Geometry: see drawing. Coordinates: mm, zero at the bounding-box minimum. Round coordinates to 2 decimals unless told otherwise and drop trailing zeros. Order: outer loops, then holes, each group sorted by start corner. A loop starts at its lowest first (then second) coordinate and runs counter-clockwise, first axis right, second up. Notation, with made-up numbers: (-26.75, -22) - (-1.75, -22) arc R26 ccw to (-1.75, 2) - close; hole circle Ø6 at (38.25, -26). An arc over 180 degrees is marked (long way). Put each result on its own line as item: value. Start each with the question number.
1) Contact query for flat-ended pins moving along their axis: P1, Ø4, axis at y = 43.5, z = 1.5, coming from the -X side; P2, Ø1, axis at y = 7.5, z = 4, coming from the -X side. Output: stop coordinate, or through.
2) Section A-A on x = 6.75. Output: boundary loops of the cut face in (y, z), then the cut area to 3 significant figures.
3) Section B-B on z = 4. Output: boundary loops of the cut face in (x, y).
4) Section C-C on y = 27. Output: boundary loops of the cut face in (x, z).
5) Line query: probe 1 along Y at (x, z) = (8.75, 7.75); probe 2 along Z at (x, y) = (2.5, 19); probe 3 along X at (y, z) = (12, 2.75). Output: solid intervals per line, ascending. Write a range as [from, to].
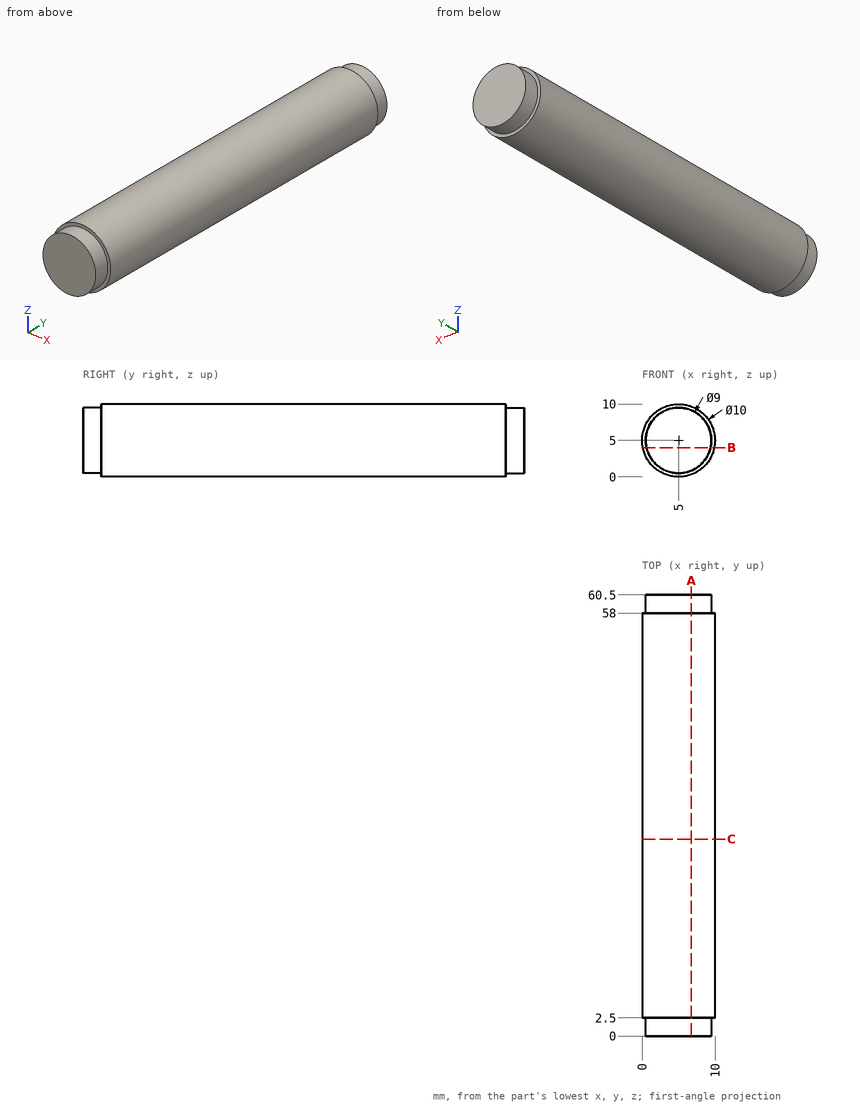
Answer sheet:
1. P1: x = 0.23
1. P2: x = 0.03
2. outline: (0, 0.85) - (2.5, 0.85) - (2.5, 0.32) - (58, 0.32) - (58, 0.85) - (60.5, 0.85) - (60.5, 9.15) - (58, 9.15) - (58, 9.68) - (2.5, 9.68) - (2.5, 9.15) - (0, 9.15) - close
2. area: 561 mm^2
3. outline: (0.1, 2.5) - (0.61, 2.5) - (0.61, 0) - (9.39, 0) - (9.39, 2.5) - (9.9, 2.5) - (9.9, 58) - (9.39, 58) - (9.39, 60.5) - (0.61, 60.5) - (0.61, 58) - (0.1, 58) - close
4. outline: circle Ø10 at (5, 5)
5. probe 1: [2.5, 58]
5. probe 2: [0.67, 9.33]
5. probe 3: [0.53, 9.47]
